The listing builds one solid part. Answer for the finished solid, in the listing's coordinates (mm). A direction names the side the tool comes from. Coordinates: 2 decimals unless noted, no trailing zeros. Order: outer loops, then holes, each group sorted by start corner. A loop starts at its lowest first (then second) coordinate and runs counter-clockwise, first axis right, second up. Notation, with made-up numbers: (22.25, 40) -> (79.25, 40) arc R3 cw to (79.25, 44) -> close; hole circle Ø7 at (80.5, 72.5). An arc over 180 degrees is marked (long way). One line per question, with ' | ' between items.
from build123d import *

# Parameters (mm, degrees)
SKETCH_1_W                   = 60
SKETCH_1_H                   = 35
EXTRUDE_1_DEPTH              = 10
HOLE_WIZARD_M4_1_D           = 4.8
HOLE_WIZARD_M4_1_CBORE_D     = 8
HOLE_WIZARD_M4_1_CBORE_DEPTH = 4
HOLE_WIZARD_M4_1_2_D         = 3.3


with BuildPart() as part:
    # 草图1 → 凸台-拉伸1 (new body)
    with BuildSketch(Plane.XY):
        with Locations((30, 17.5)):
            Rectangle(SKETCH_1_W, SKETCH_1_H)
    extrude(amount=EXTRUDE_1_DEPTH)

    # Hole Wizard M4 _1 (through all)
    with Locations(Plane(origin=(0, 0, 0), x_dir=(-1, 0, 0), z_dir=(0, 0, -1))):
        with Locations((-55, 7.5), (-55, 27.5)):
            CounterBoreHole(HOLE_WIZARD_M4_1_D / 2, HOLE_WIZARD_M4_1_CBORE_D / 2, HOLE_WIZARD_M4_1_CBORE_DEPTH)

    # Hole Wizard M4 _1 2 (through all)
    with Locations(Plane(origin=(0, 0, 0), x_dir=(-1, 0, 0), z_dir=(0, 0, -1))):
        with Locations((-22, 25), (-22, 15)):
            Hole(HOLE_WIZARD_M4_1_2_D / 2)


solid = part.part
Item 1: Determine the mould class of faces 3 (the face through (60, 17, 5)), 4 (the face through (30, 18, 0)), 5 (the face through (0, 17, 5)), 6 (the face through (51.185, 8.701, 1.972)) for opening direction X: pulls with the +X half, pulls with the -X half, needs draft (parallel to the pull), parting line crosses it, or undercut.
Computed values:
face 3: pulls with the +X half | face 4: needs draft | face 5: pulls with the -X half | face 6: undercut
Item 2: Section A-A, the plane x = 55 is taken. Give the vertices of the cut face in (y, z), plus the area to 3 significant figures.
Computed values:
outline: (0, 0) -> (3.5, 0) -> (3.5, 4) -> (5.1, 4) -> (5.1, 10) -> (0, 10) -> close; (9.9, 4) -> (11.5, 4) -> (11.5, 0) -> (23.5, 0) -> (23.5, 4) -> (25.1, 4) -> (25.1, 10) -> (9.9, 10) -> close; (29.9, 4) -> (31.5, 4) -> (31.5, 0) -> (35, 0) -> (35, 10) -> (29.9, 10) -> close | area: 228 mm^2
Item 3: Section D-D, the plane y = 15 is taken. Give the vertices of the cut face in (x, z), plus the area to 3 significant figures.
Computed values:
outline: (0, 0) -> (20.35, 0) -> (20.35, 10) -> (0, 10) -> close; (23.65, 0) -> (60, 0) -> (60, 10) -> (23.65, 10) -> close | area: 567 mm^2
Item 4: Section B-B, the plane y = 27.5 is taken. Give the vertices of the cut face in (x, z).
Computed values:
outline: (0, 0) -> (51, 0) -> (51, 4) -> (52.6, 4) -> (52.6, 10) -> (0, 10) -> close; (57.4, 4) -> (59, 4) -> (59, 0) -> (60, 0) -> (60, 10) -> (57.4, 10) -> close
Item 5: Each of these flat-tipped pins is pushed along its axis until it touches: pin 1 Ø2.5 at (x, y) = (53, 26.5) entering from -Z; pin 2 Ø2 at (x, y) = (22, 15) entering from -Z. Where does it stop, or does it pass through?
Computed values:
pin 1: stops at z = 4 | pin 2: passes through
Item 6: For faces 1 (the face through (55.1, 4.9, 4)), 2 (the face through (56.11, 25.37, 7.04)), determine the directions among +Z, -Z, +X, -X, +Y, -Y from which every point of the face is accessible in a straight line to the end or side of a thin tool.
Computed values:
face 1: -Z | face 2: +Z, -Z
Item 7: Section C-C, the plane z = 2.5 is taken. Give the vertices of the cut face in (x, y), plus the area to 3 significant figures.
Computed values:
outline: (0, 0) -> (60, 0) -> (60, 35) -> (0, 35) -> close; hole circle Ø3.3 at (22, 15); hole circle Ø3.3 at (22, 25); hole circle Ø8 at (55, 7.5); hole circle Ø8 at (55, 27.5) | area: 1,980 mm^2
Item 8: Find the intervals of material crossed by L1, parallel to Y at x = 55, z = 6.05; L2, parallel to Y at x = 23, z = 7.75; L3, parallel to X at y = 7, z = 2, in increasing order.
Computed values:
L1: y = 0 to 5.1, 9.9 to 25.1, 29.9 to 35 | L2: y = 0 to 13.69, 16.31 to 23.69, 26.31 to 35 | L3: x = 0 to 51.03, 58.97 to 60
